The model under review builds one solid part; all positions refer to its coordinate system, in mm. A direction names the side the tool comes from. Coordinates: 2 decimals unless noted, no trailing zeros. Write each loop counter-clockwise with the first axis right and the second up, starting at its lowest first coordinate (ties: lowest second). Pieces come first, ordered by that corner, then holes. Notation, with made-up numbers: (27, -18.5) - (85, -18.5) arc R4 cw to (85, -11.5) - close; hole circle Ø4 at (-4.5, -12). An arc over 180 degrees is marked (long way). Put each result on its own line as item: value.
from build123d import *

# Parameters (mm, degrees)
F0_W     = 46.2
F0_H     = 46.2
F1_DEPTH = 116
F0_W_2   = 60
F0_H_2   = 60
F2_DEPTH = 4
F3_R     = 4
F4_R     = 2
F7_DEPTH = 80


with BuildPart() as f1:
    # F0 (on Top) → F1 (new body)
    with BuildSketch(Plane.XY):
        Polygon((27.65, 17.65), (27.65, 27.65), (-27.65, 27.65), (-27.65, 17.65), (-28.05, 17.65), (-28.05, 7.65), (-27.65, 7.65), (-27.65, -7.65), (-28.05, -7.65), (-28.05, -17.65), (-27.65, -17.65), (-27.65, -27.65), (-17.65, -27.65), (-17.65, -27.95), (-7.65, -27.95), (-7.65, -27.65), (7.65, -27.65), (7.65, -27.95), (17.65, -27.95), (17.65, -27.65), (27.65, -27.65), (27.65, -17.65), (28.05, -17.65), (28.05, -7.65), (27.65, -7.65), (27.65, 7.65), (28.05, 7.65), (28.05, 17.65), align=None)
        Rectangle(F0_W, F0_H, mode=Mode.SUBTRACT)
    extrude(amount=F1_DEPTH)

    # F0 (on Top) → F2 (join)
    with BuildSketch(Plane.XY):
        Rectangle(F0_W_2, F0_H_2)
        Polygon((-27.65, 27.65), (27.65, 27.65), (27.65, 17.65), (28.05, 17.65), (28.05, 7.65), (27.65, 7.65), (27.65, -7.65), (28.05, -7.65), (28.05, -17.65), (27.65, -17.65), (27.65, -27.65), (17.65, -27.65), (17.65, -27.95), (7.65, -27.95), (7.65, -27.65), (-7.65, -27.65), (-7.65, -27.95), (-17.65, -27.95), (-17.65, -27.65), (-27.65, -27.65), (-27.65, -17.65), (-28.05, -17.65), (-28.05, -7.65), (-27.65, -7.65), (-27.65, 7.65), (-28.05, 7.65), (-28.05, 17.65), (-27.65, 17.65), align=None, mode=Mode.SUBTRACT)
        Polygon((27.65, 17.65), (27.65, 27.65), (-27.65, 27.65), (-27.65, 17.65), (-28.05, 17.65), (-28.05, 7.65), (-27.65, 7.65), (-27.65, -7.65), (-28.05, -7.65), (-28.05, -17.65), (-27.65, -17.65), (-27.65, -27.65), (-17.65, -27.65), (-17.65, -27.95), (-7.65, -27.95), (-7.65, -27.65), (7.65, -27.65), (7.65, -27.95), (17.65, -27.95), (17.65, -27.65), (27.65, -27.65), (27.65, -17.65), (28.05, -17.65), (28.05, -7.65), (27.65, -7.65), (27.65, 7.65), (28.05, 7.65), (28.05, 17.65), align=None)
        Rectangle(F0_W, F0_H, mode=Mode.SUBTRACT)
    extrude(amount=-F2_DEPTH)

    # F3
    f3_edges = [f1.edges().sort_by_distance(p)[0] for p in [
        (27.65, -27.65, 58),
        (-27.65, -27.65, 58),
        (27.65, 27.65, 58),
        (-27.65, 27.65, 58),
        (-30, 30, -2),
        (30, 30, -2),
        (-30, -30, -2),
        (30, -30, -2),
    ]]
    fillet(f3_edges, radius=F3_R)

    # F4
    f4_edges = [f1.edges().sort_by_distance(p)[0] for p in [
        (30, 0, -4),
    ]]
    fillet(f4_edges, radius=F4_R)

    # F6 (on offset) → F7 (cut)
    with BuildSketch(Plane.XZ.offset(27.65)):
        with BuildLine():
            Line((-5.630705, 67.75), (-7.370688, 62.394882))
            ThreePointArc((-7.370688, 62.394882), (0, 52.25), (7.370688, 62.394882))
            Line((7.370688, 62.394882), (5.630705, 67.75))
            Line((5.630705, 67.75), (-5.630705, 67.75))
        make_face()
    extrude(amount=-F7_DEPTH, mode=Mode.SUBTRACT)


solid = f1.part
1. Consider section C-C on x = 0. State the section outline as (y, z) points, plus the area to 3 significant figures.
Determined:
outline: (-30, -2) arc R2 ccw to (-28, -4) - (-23.1, -4) - (-23.1, 52.25) - (-27.65, 52.25) - (-27.65, 0) - (-30, 0) - close; (-27.65, 67.75) - (-23.1, 67.75) - (-23.1, 116) - (-27.65, 116) - close; (23.1, -4) - (28, -4) arc R2 ccw to (30, -2) - (30, 0) - (27.65, 0) - (27.65, 52.25) - (23.1, 52.25) - close; (23.1, 67.75) - (27.65, 67.75) - (27.65, 116) - (23.1, 116) - close
area: 968 mm^2
2. To check wall thickness, follow probe 1 along Y at (x, z) = (18, 44.5); probe 2 along Y at (x, z) = (-9, 7). State the ranges of each line that lie inside material, in increasing order.
Determined:
probe 1: y = -27.65 to -23.1, 23.1 to 27.65
probe 2: y = -27.95 to -23.1, 23.1 to 27.65
3. Machinability: for faces 1 (the cylindrical face through (26.447, 26.509, 58.812)), 2 (the flat face through (21, -27.65, 57)), 3 (the flat face through (-6.49, -25.41, 65.11)), 4 (the cylindrical face through (-26.509, 26.447, 58.812)), which of the approach directions +Z, -Z, +X, -X, +Y, -Y give a long, thin tool a straight path to every point of the face, cutting with its end or side? Answer none if there is none.
Determined:
face 1: +Z, +X, +Y
face 2: +Z, +X, -Y
face 3: +Y, -Y
face 4: +Z, -X, +Y
4. For pin 1 Ø5 at (x, z) = (17, 21.5) entering from +Y; pin 2 Ø1 at (x, z) = (16, 40) entering from -Y; pin 3 Ø7.5 at (y, z) = (3, 47) entering from +X, all flat-tipped, find the tip position at first contact; note any pin that passes through.
Determined:
pin 1: stops at y = 27.65
pin 2: stops at y = -27.95
pin 3: stops at x = 27.65
5. The part is to be moulded in two halves that separate along X. For faces 5 (the flat face through (-27.65, 21, 57)), 6 (the flat face through (-23.1, 0, 57)), 7 (the cylindrical face through (28.859, -28.797, -1.014)), 8 (the cylindrical face through (-0.204, 25.343, 52.253)), say which applies: +X half, -X half, draft (parallel to the pull), parting line (faces both ways), or undercut.
Determined:
face 5: -X half
face 6: undercut
face 7: +X half
face 8: undercut
6. Consider section A-A on x = 19. State the section outline as (y, z) points, plus the area to 3 significant figures.
Determined:
outline: (-30, -2) arc R2 ccw to (-28, -4) - (-23.1, -4) - (-23.1, 116) - (-27.65, 116) - (-27.65, 0) - (-30, 0) - close; (23.1, -4) - (28, -4) arc R2 ccw to (30, -2) - (30, 0) - (27.65, 0) - (27.65, 116) - (23.1, 116) - close
area: 1,110 mm^2
